Build history of the part. All positions in model axes, mm. Round coordinates to 2 decimals unless told otherwise and drop trailing zeros. Write each loop counter-clockwise with the first axis right and the second up, starting at its lowest first coordinate (ties: lowest second). Pieces come first, ordered by that corner, then holes.
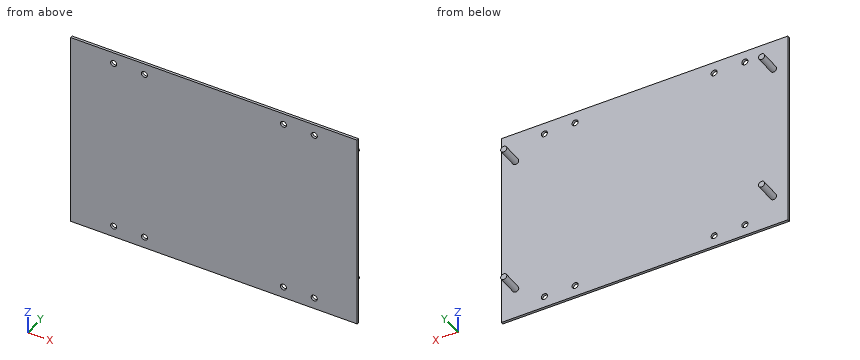
from build123d import *

# Parameters (mm, degrees)
SKETCH1_W           = 139.7
SKETCH1_H           = 98.044
SKETCH1_R           = 1.5
BOSS_EXTRUDE1_DEPTH = 1.2
SKETCH2_R           = 1.5
BOSS_EXTRUDE2_DEPTH = 10


with BuildPart() as part:
    # Sketch1 → Boss-Extrude1 (new body)
    with BuildSketch(Plane(origin=(0, 0, 0), x_dir=(1, 0, 0), z_dir=(0, 1, 0))):
        with Locations((0, 3.302)):
            Rectangle(SKETCH1_W, SKETCH1_H)
        with Locations(Location((-48.8772454, -40.12, 0), (0, 0, 270))):
            Circle(SKETCH1_R, mode=Mode.SUBTRACT)
        with Locations(Location((-33.8772454, -40.12, 0), (0, 0, 270))):
            Circle(SKETCH1_R, mode=Mode.SUBTRACT)
        with Locations(Location((-33.891248194, 46.724, 0), (0, 0, 90))):
            Circle(SKETCH1_R, mode=Mode.SUBTRACT)
        with Locations(Location((-48.877248194, 46.724, 0), (0, 0, 90))):
            Circle(SKETCH1_R, mode=Mode.SUBTRACT)
        with Locations(Location((33.878607802, 46.724, 0), (0, 0, 270))):
            Circle(SKETCH1_R, mode=Mode.SUBTRACT)
        with Locations(Location((48.8772454, 46.724, 0), (0, 0, 270))):
            Circle(SKETCH1_R, mode=Mode.SUBTRACT)
        with Locations(Location((33.8772454, -40.12, 0), (0, 0, 90))):
            Circle(SKETCH1_R, mode=Mode.SUBTRACT)
        with Locations(Location((48.8772454, -40.12, 0), (0, 0, 90))):
            Circle(SKETCH1_R, mode=Mode.SUBTRACT)
    extrude(amount=BOSS_EXTRUDE1_DEPTH)

    # Sketch2 → Boss-Extrude2 (add)
    with BuildSketch(Plane(origin=(0, 1.2, 0), x_dir=(1, 0, 0), z_dir=(0, 1, 0))):
        with Locations(Location((-62.85, 37.324, 0), (0, 0, 90))):
            Circle(SKETCH2_R)
        with Locations(Location((-62.85, -30.72, 0), (0, 0, 90))):
            Circle(SKETCH2_R)
        with Locations(Location((62.85, -30.72, 0), (0, 0, 90))):
            Circle(SKETCH2_R)
        with Locations(Location((62.85, 37.324, 0), (0, 0, 90))):
            Circle(SKETCH2_R)
    extrude(amount=BOSS_EXTRUDE2_DEPTH)


solid = part.part
1) Slice it at A-A (z = 40.12). Write the cut outline in (x, y), plus the area to 3 significant figures.
Results:
outline: (-69.85, 0) - (-50.38, 0) - (-50.38, 1.2) - (-69.85, 1.2) - close; (-47.38, 0) - (-35.38, 0) - (-35.38, 1.2) - (-47.38, 1.2) - close; (-32.38, 0) - (32.38, 0) - (32.38, 1.2) - (-32.38, 1.2) - close; (35.38, 0) - (47.38, 0) - (47.38, 1.2) - (35.38, 1.2) - close; (50.38, 0) - (69.85, 0) - (69.85, 1.2) - (50.38, 1.2) - close
area: 153 mm2
2) Wall check: L1, parallel to X at y = 0.95, z = 40.12; L2, parallel to Y at x = 4.5, z = 24. Give the ranges that are in metal, low to high.
Results:
L1: x = -69.85 to -50.38, -47.38 to -35.38, -32.38 to 32.38, 35.38 to 47.38, 50.38 to 69.85
L2: y = 0 to 1.2
3) Slice it at D-D (x = -10). Write the cut outline in (y, z), plus the area to 3 significant figures.
Results:
outline: (0, -52.32) - (1.2, -52.32) - (1.2, 45.72) - (0, 45.72) - close
area: 118 mm2
4) Slice it at B-B (x = -62.85). Write the cut outline in (y, z).
Results:
outline: (0, -52.32) - (1.2, -52.32) - (1.2, -38.82) - (11.2, -38.82) - (11.2, -35.82) - (1.2, -35.82) - (1.2, 29.22) - (11.2, 29.22) - (11.2, 32.22) - (1.2, 32.22) - (1.2, 45.72) - (0, 45.72) - close
5) Slice it at C-C (y = 8.5). Write the cut outline in (x, z), plus the area to 3 significant figures.
Results:
outline: circle Ø3 at (-62.85, -37.32); circle Ø3 at (-62.85, 30.72); circle Ø3 at (62.85, -37.32); circle Ø3 at (62.85, 30.72)
area: 28.3 mm2
6) Pin check, flat tips, straight feed: pin 1 Ø3 at (x, y) = (23, 2.5) entering from -Z; pin 2 Ø6 at (y, z) = (7, 30.5) entering from -X; pin 3 Ø3.5 at (x, z) = (33.88, -46.72) entering from +Y. Stop position of each tip, or through.
Results:
pin 1: stops at z = -52.32
pin 2: stops at x = -64.35
pin 3: stops at y = 1.2
